For this review, take the finished solid that the model builds, in its own axes (mm). A direction names the side the tool comes from. Coordinates: 2 decimals unless noted, no trailing zeros. Order: outer loops, then holes, each group sorted by start corner. A loop starts at its lowest first (then second) coordinate and runs counter-clockwise, first axis right, second up. Notation, with made-up numbers: (72, 86.25) -> (100, 86.25) arc R34 ccw to (100, 116.25) -> close; hole circle Ø9 at (-21.5, -32). An arc over 180 degrees is marked (long way). Answer as a JSON object with one key per item and string values. Group by question number.
1) Draft analysis for pull direction Z (two halves, no side actions). For faces 1 (the flat face through (66.108, 1, -12)), 2 (the flat face through (38, 0, -24)), 3 (the flat face through (38, 1, -48)), state which applies: +Z half, -Z half, draft (parallel to the pull), parting line (faces both ways), or undercut.
2) Add section C-C, the plane x = 21. Write out the cut boundary in (y, z).
3) Add section D-D, the plane z = -40. Write out the cut boundary in (x, y).
4) Machinability: for faces 4 (the flat face through (57.108, 1, -12)), 5 (the flat face through (38, 1, 0)), which of the approach directions +Z, -Z, +X, -X, +Y, -Y give a long, thin tool a straight path to every point of the face, cutting with its end or side? Answer none if there is none.
5) Add section B-B, the plane y = 1.65. Write out the cut boundary in (x, z), then the cut area to 3 significant figures.
6) Add section A-A, the plane z = -28. Write out the cut boundary in (x, y).
7) For pin 1 (8.5 mm diameter, centred on x = 21, z = -28, fed in from -Y); pin 2 (0.5 mm diameter, centred on x = 0.5, z = -22.5, fed in from +Y); pin 3 (0.6 mm diameter, centred on y = 1.5, z = -12.5, fed in from +X), all flat-tipped, find the tip position at first contact; note any pin that passes through.
8) Wall thickness on L1, parallel to X at y = 1.4, z = -10; L2, parallel to Z at x = 70.5, y = 0.9; L3, parallel to X at y = 0.7, z = -10: over which ranges is each line inside the solid? List them lowest first.
from build123d import *

# Parameters (mm, degrees)
SKETCH1_W              = 77.5
SKETCH1_H              = 48
BOSS_EXTRUDE1_DEPTH    = 2
SKETCH2_W              = 1
SKETCH2_H              = 48
CUT_EXTRUDE1_DEPTH     = 1.2
SKETCH3_R              = 4
CUT_EXTRUDE2_DEPTH     = 2
SKETCH4_R              = 1.5
SKETCH4_W              = 9
SKETCH4_H              = 14
CUT_EXTRUDE3_DEPTH     = 12
CUT_EXTRUDE4_OUTLINE_R = 4.75
CUT_EXTRUDE4_DEPTH     = 2


# Read off the part's stored shape, not the designer's step: Cut-Extrude4
with BuildPart() as part:
    # Sketch1 → Boss-Extrude1 (new body)
    with BuildSketch(Plane(origin=(0, 0, 0), x_dir=(1, 0, 0), z_dir=(0, 1, 0))):
        with Locations((38.75, 24)):
            Rectangle(SKETCH1_W, SKETCH1_H)
    extrude(amount=BOSS_EXTRUDE1_DEPTH)

    # Sketch2 → Cut-Extrude1 (cut)
    with BuildSketch(Plane(origin=(0, 2, 0), x_dir=(1, 0, 0), z_dir=(0, 1, 0))):
        with Locations((0.5, 24)):
            Rectangle(SKETCH2_W, SKETCH2_H)
        with Locations((77, 24)):
            Rectangle(SKETCH2_W, SKETCH2_H)
    extrude(amount=-CUT_EXTRUDE1_DEPTH, mode=Mode.SUBTRACT)

    # Sketch3 → Cut-Extrude2 (cut)
    with BuildSketch(Plane(origin=(0, 2, 0), x_dir=(1, 0, 0), z_dir=(0, 1, 0))):
        with Locations(Location((22, 10, 0), (0, 0, 270))):
            Circle(SKETCH3_R)
    extrude(amount=-CUT_EXTRUDE2_DEPTH, mode=Mode.SUBTRACT)

    # Sketch4 → Cut-Extrude3 (cut)
    with BuildSketch(Plane(origin=(0, 2, 0), x_dir=(1, 0, 0), z_dir=(0, 1, 0))):
        with Locations(Location((70.5, 7, 0), (0, 0, 270))):
            Circle(SKETCH4_R)
        with Locations((61.608422626, 12.013032017)):
            Rectangle(SKETCH4_W, SKETCH4_H)
    extrude(amount=-CUT_EXTRUDE3_DEPTH, mode=Mode.SUBTRACT)

    # Cut-Extrude4 outline → Cut-Extrude4 (cut)
    with BuildSketch(Plane(origin=(0, 0, 0), x_dir=(1, 0, 0), z_dir=(0, 1, 0))):
        with Locations((21, 28)):
            Circle(CUT_EXTRUDE4_OUTLINE_R)
    extrude(amount=CUT_EXTRUDE4_DEPTH, mode=Mode.SUBTRACT)


solid = part.part
Output values:
{
 "1": {"face 1": "undercut", "face 2": "draft", "face 3": "-Z half"},
 "2": {"outline": "(0, -48) -> (2, -48) -> (2, -32.75) -> (0, -32.75) -> close; (0, -23.25) -> (2, -23.25) -> (2, -13.87) -> (0, -13.87) -> close; (0, -6.13) -> (2, -6.13) -> (2, 0) -> (0, 0) -> close"},
 "3": {"outline": "(0, 0) -> (77.5, 0) -> (77.5, 0.8) -> (76.5, 0.8) -> (76.5, 2) -> (1, 2) -> (1, 0.8) -> (0, 0.8) -> close"},
 "4": {"face 4": "+Y, -Y", "face 5": "+Z, +X, -X, +Y, -Y"},
 "5": {"outline": "(1, -48) -> (76.5, -48) -> (76.5, 0) -> (1, 0) -> close; hole circle Ø9.5 at (21, -28); hole circle Ø8 at (22, -10); hole (57.11, -19.01) -> (66.11, -19.01) -> (66.11, -5.01) -> (57.11, -5.01) -> close; hole circle Ø3 at (70.5, -7)", "area": "3,370 mm²"},
 "6": {"outline": "(0, 0) -> (16.25, 0) -> (16.25, 2) -> (1, 2) -> (1, 0.8) -> (0, 0.8) -> close; (25.75, 0) -> (77.5, 0) -> (77.5, 0.8) -> (76.5, 0.8) -> (76.5, 2) -> (25.75, 2) -> close"},
 "7": {"pin 1": "passes through", "pin 2": "stops at y = 0.8", "pin 3": "stops at x = 76.5"},
 "8": {"L1": "x = 1 to 18, 26 to 57.11, 66.11 to 76.5", "L2": "z = -48 to -8.5, -5.5 to 0", "L3": "x = 0 to 18, 26 to 57.11, 66.11 to 77.5"}
}
